```python
from build123d import *

# Parameters (mm, degrees)
SALIENTE_EXTRUIR1_DEPTH = 30
CORTAR_EXTRUIR1_START   = -12
CORTAR_EXTRUIR1_DEPTH   = 12
CORTAR_EXTRUIR2_REACH   = 35.679
CROQUIS3_R              = 1.65


# Read off the part's stored shape, not the designer's step: Cortar-Extruir1
with BuildPart() as part:
    # Croquis1 → Saliente-Extruir1 (new body)
    with BuildSketch(Plane.XY):
        Polygon((12, 0), (12, 12.5), (7, 12.5), (7, 3), (0, 3), (0, 0), align=None)
    extrude(amount=SALIENTE_EXTRUIR1_DEPTH)

    # Cortar-Extruir1 outline → Cortar-Extruir1 (cut)
    with BuildSketch(Plane(origin=(0, 12.5, 0), x_dir=(1, 0, 0), z_dir=(0, 1, 0)).offset(CORTAR_EXTRUIR1_START)):
        Polygon((12, -23.1), (12, -6.1), (11, -6.1), (11, -4.1), (8.96, -4.1), (8.96, -25.1), (11, -25.1), (11, -23.1), align=None)
    extrude(amount=CORTAR_EXTRUIR1_DEPTH, mode=Mode.SUBTRACT)

    # Croquis3 → Cortar-Extruir2 (cut, up to next)
    with BuildSketch(Plane(origin=(0, 3, 0), x_dir=(1, 0, 0), z_dir=(0, 1, 0)), mode=Mode.PRIVATE) as cortar_extruir2_sk1:
        with Locations(Location((3.5, -6, 0), (0, 0, 270))):
            Circle(CROQUIS3_R)
    cortar_extruir2_tool1 = extrude(cortar_extruir2_sk1.sketch, amount=-CORTAR_EXTRUIR2_REACH, mode=Mode.PRIVATE) & part.part
    # Croquis3 → Cortar-Extruir2 (cut, up to next)
    with BuildSketch(Plane(origin=(0, 3, 0), x_dir=(1, 0, 0), z_dir=(0, 1, 0)), mode=Mode.PRIVATE) as cortar_extruir2_sk2:
        with Locations(Location((3.5, -24, 0), (0, 0, 270))):
            Circle(CROQUIS3_R)
    cortar_extruir2_tool2 = extrude(cortar_extruir2_sk2.sketch, amount=-CORTAR_EXTRUIR2_REACH, mode=Mode.PRIVATE) & part.part
    add(cortar_extruir2_tool1.solids().sort_by_distance((3.5, 3, 6))[0], mode=Mode.SUBTRACT)
    add(cortar_extruir2_tool2.solids().sort_by_distance((3.5, 3, 24))[0], mode=Mode.SUBTRACT)


solid = part.part
```
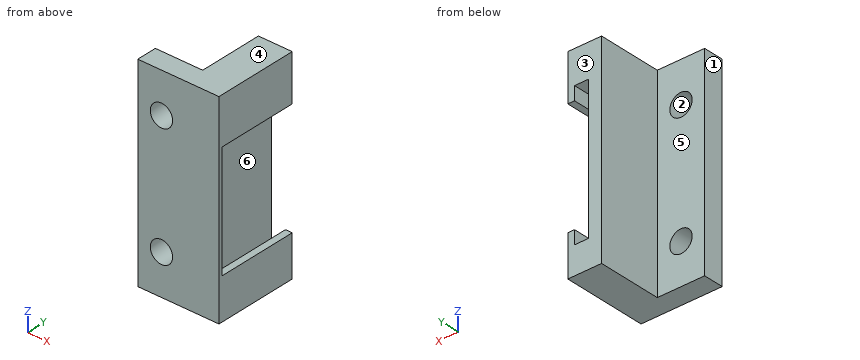
The listing builds one solid part. Answer for the finished solid, in the listing's coordinates (mm). Face numbers are marked on the shaded views. A direction names the side the tool comes from. Give positions to 0.01 mm unless a question says otherwise; leave off trailing zeros. Order: outer loops, then holes, each group sorted by start corner. A loop starts at its lowest first (then second) coordinate and runs counter-clockwise, first axis right, second up.
1) Given P1, Ø3.5, axis at y = 6, z = 11.5, coming from the +X side; P2, Ø2, axis at x = 3.5, z = 9.5, coming from the +Y side; P3, Ø3, axis at x = 3.5, z = 24, coming from the -Y side; P4, Ø1.6, axis at y = 5.5, z = 5.5, coming from the -X side, each flat-ended and moving along its own axis, determine where each tip first touches the part or whether it passes through.
Reported:
P1: stops at x = 8.96
P2: stops at y = 3
P3: passes through
P4: stops at x = 7
2) Consider line 1 along X through (y, z) = (1.7, 6); line 2 along X through (y, z) = (12.25, 23.25); line 3 along Z through (x, y) = (2.5, 2). Determine where each line is inside the solid, lowest interval first.
Reported:
line 1: x = 0 to 1.85, 5.15 to 8.96, 11 to 12
line 2: x = 7 to 8.96, 11 to 12
line 3: z = 0 to 4.69, 7.31 to 22.69, 25.31 to 30
3) Determine the mould class of the marked faces 1, 2 and 3 for opening direction X: pulls with the +X half, pulls with the -X half, needs draft (parallel to the pull), parting line crosses it, or undercut.
Reported:
face 1: pulls with the -X half
face 2: undercut
face 3: needs draft
4) Find section D-D on x = 9.5. Write down the section's boundary in (y, z), then the cut area to 3 significant figures.
Reported:
outline: (0, 0) - (12.5, 0) - (12.5, 4.1) - (0.5, 4.1) - (0.5, 25.1) - (12.5, 25.1) - (12.5, 30) - (0, 30) - close
area: 123 mm2
5) Find section C-C on y = 10.75. Write down the section's boundary in (x, z), then the cut area to 3 significant figures.
Reported:
outline: (7, 0) - (12, 0) - (12, 6.1) - (11, 6.1) - (11, 4.1) - (8.96, 4.1) - (8.96, 25.1) - (11, 25.1) - (11, 23.1) - (12, 23.1) - (12, 30) - (7, 30) - close
area: 90.2 mm2
6) For the marked faces 4, 5 and 6, determine the directions among +Z, -Z, +X, -X, +Y, -Y from which every point of the face is accessible in a straight line to the end or side of a thin tool.
Reported:
face 4: +Z, +X, -X, +Y, -Y
face 5: +Z, -Z, -X, +Y
face 6: +Y
7) Find section B-B on x = 3.5. Write down the section's boundary in (y, z), then the cut area to 3 significant figures.
Reported:
outline: (0, 0) - (3, 0) - (3, 4.35) - (0, 4.35) - close; (0, 7.65) - (3, 7.65) - (3, 22.35) - (0, 22.35) - close; (0, 25.65) - (3, 25.65) - (3, 30) - (0, 30) - close
area: 70.2 mm2
8) Find section A-A on z = 24. Write down the section's boundary in (x, y).
Reported:
outline: (0, 0) - (1.85, 0) - (1.85, 3) - (0, 3) - close; (5.15, 0) - (12, 0) - (12, 12.5) - (11, 12.5) - (11, 0.5) - (8.96, 0.5) - (8.96, 12.5) - (7, 12.5) - (7, 3) - (5.15, 3) - close
